from build123d import *

# Parameters (mm, degrees)
F1_DEPTH = 25.4


with BuildPart() as f1:
    # F0 (on Front) → F1 (new body)
    with BuildSketch(Plane.XZ):
        with BuildLine():
            ThreePointArc((14.261975499, -21.0179935975), (-24.2797965125, -7.459992045), (0, 25.4))
            Line((0, 25.4), (0, 39.37))
            add(Edge.make_bspline(
                [(0, 39.37), (-19.553380087, 37.3347476125), (-45.5671340259, -1.5697728715), (-8.319397981, -32.2288283909), (10.069599463, -24.265725606), (14.261975499, -21.0179935975)],
                knots=[0, 0, 0, 0, 0.2762654828, 0.5259592689, 0.6180466386, 0.6180466386, 0.6180466386, 0.6180466386], degree=3))
        make_face()
        with BuildLine():
            ThreePointArc((23.4435268904, -9.7755330769), (24.9060794086, -4.9846974323), (25.4, 0))
            ThreePointArc((25.4, 0), (18.8885688435, 16.9818128315), (2.6927585006, 25.2568614768))
            add(Edge.make_bspline(
                [(2.6927585006, 25.2568614768), (1.8135864389, 25.3433698488), (0.9156429342, 25.3918395582), (0, 25.4)],
                knots=[0.9865811397, 0.9865811397, 0.9865811397, 0.9865811397, 1, 1, 1, 1], degree=3))
            ThreePointArc((0, 25.4), (-24.2797965125, -7.459992045), (14.261975499, -21.0179935975))
            add(Edge.make_bspline(
                [(14.261975499, -21.0179935975), (18.1280082, -18.0230718536), (21.3458508833, -14.0908635275), (23.4435268904, -9.7755330769)],
                knots=[0.6180466386, 0.6180466386, 0.6180466386, 0.6180466386, 0.7029657344, 0.7029657344, 0.7029657344, 0.7029657344], degree=3))
        make_face()
    extrude(amount=F1_DEPTH)


solid = f1.part
The listing builds one solid part. Answer for the finished solid, in the listing's coordinates (mm). A direction names the side the tool comes from. Coordinates: 2 decimals unless noted, no trailing zeros. Answer in a Markdown table with one row per item. Add a question column.
Item 1: Each of these flat-tipped pins is pushed along its axis until it touches: P1, Ø7, axis at y = -8.5, z = 29, coming from the +X side; P2, Ø3, axis at x = 13, y = -21.5, coming from the -Z side; P3, Ø5, axis at x = 18, y = -11, coming from the -Z side. Where does it stop, or does it pass through?
Item 2: Which of the six approach directions +Z, -Z, +X, -X, +Y, -Y give full straight-line access (tool end or side, diameter ignored) to faces 1 (the face through (-3, -25.4, 4)), 2 (the face through (0, -13, 32))?
Item 3: Find the intervals of material crossed by L1, parallel to X at y = -16.75, z = -4; L2, parallel to Z at x = 1.5, y = -18; L3, parallel to Z at x = -14.5, y = -6.5, in increasing order. Write a range as from..to.
Result set:
| question | item | result |
|---|---|---|
| 1 | P1 | stops at x = 0 |
| 1 | P2 | stops at z = -22.93 |
| 1 | P3 | stops at z = -20.01 |
| 2 | face 1 | +Z, -Z, +X, -X, -Y |
| 2 | face 2 | +Z, +X, +Y, -Y |
| 3 | L1 | x = -30.12..25.08 |
| 3 | L2 | z = -26.6..25.35 |
| 3 | L3 | z = -23.2..34.03 |
